```python
from build123d import *

# Parameters (mm, degrees)
BOSS_EXTRUDE1_DEPTH = 10
FILLET1_R           = 10
FILLET2_R           = 10


with BuildPart() as part:
    # Sketch2 → Boss-Extrude1 (new body)
    with BuildSketch(Plane.XY):
        Polygon((-10.989010989, 64.197802198), (29.010989011, 64.197802198), (29.010989011, -37.802197802), (-5.989010989, -37.802197802), align=None)
    extrude(amount=BOSS_EXTRUDE1_DEPTH)

    # Fillet1
    # the kernel refuses this fillet: 10 mm, written as the material it takes off along each edge
    with BuildSketch(Plane(origin=(-35.989010989, 64.197802198, 0), x_dir=(0, 0, 1), z_dir=(1, 0, 0))) as fillet1_piece_1:
        with BuildLine():
            CenterArc((FILLET1_R, FILLET1_R), FILLET1_R, 180, 90)
            Line((0, FILLET1_R), (0, 0))
            Line((0, 0), (FILLET1_R, 0))
        make_face()
    extrude(amount=90, mode=Mode.SUBTRACT)
    with BuildSketch(Plane(origin=(-35.989010989, 64.197802198, 10), x_dir=(0, 0, -1), z_dir=(1, 0, 0))) as fillet1_piece_2:
        with BuildLine():
            CenterArc((FILLET1_R, -FILLET1_R), FILLET1_R, 90, 90)
            Line((0, -FILLET1_R), (0, 0))
            Line((0, 0), (FILLET1_R, 0))
        make_face()
    extrude(amount=90, mode=Mode.SUBTRACT)

    # Fillet2
    # the kernel refuses this fillet: 10 mm, written as the material it takes off along each edge
    with BuildSketch(Plane(origin=(54.010989011, -37.802197802, 0), x_dir=(0, 0, 1), z_dir=(-1, 0, 0)), Plane(origin=(54.010989011, -37.802197802, 10), x_dir=(0, 1, 0), z_dir=(-1, 0, 0))) as fillet2_piece_1:
        with BuildLine():
            CenterArc((FILLET2_R, FILLET2_R), FILLET2_R, 180, 90)
            Line((0, FILLET2_R), (0, 0))
            Line((0, 0), (FILLET2_R, 0))
        make_face()
    extrude(amount=85, mode=Mode.SUBTRACT)


solid = part.part
```
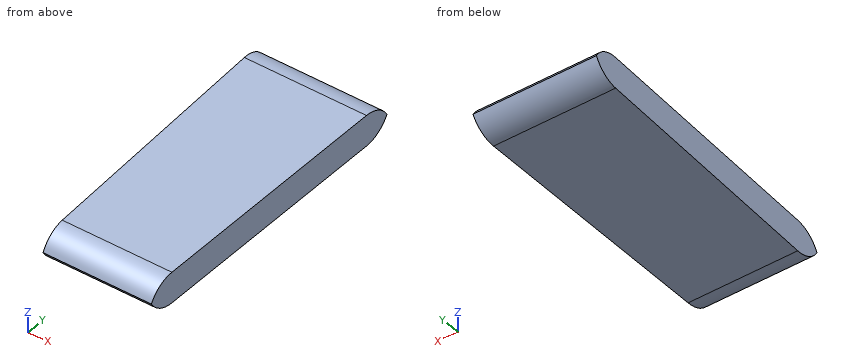
Can you work these out from the model? Positions are in its coordinate system, mm. Round coordinates to 2 decimals unless told otherwise and drop trailing zeros. Order: outer loops, then holes, each group sorted by start corner. A loop starts at its lowest first (then second) coordinate and runs counter-clockwise, first axis right, second up. Notation, with made-up numbers: (85.25, 61) -> (114.25, 61) arc R14 cw to (114.25, 66) -> close; hole circle Ø1 at (43.25, 58). An arc over 180 degrees is marked (long way). Return JSON: item names as keys, results as strings. Group by question number.
1. I need wall thicknesses on line 1 (X direction, y = 54.5, z = 3.5); line 2 (Y direction, x = 9, z = 2); line 3 (Y direction, x = 6, z = 3.75). Which ranges of each line are inside material? Lowest first, please. Write a range as [from, to].
2. Will these pins go through, and if not, where does the flat tip stop? pin 1 (4 mm diameter, centred on y = 0, z = 6.5, fed in from -X); pin 2 (1.5 mm diameter, centred on y = -16.5, z = 2.5, fed in from -X).
3. If we section it at B-B, the plane y = 28: Write out the boundary of the cut face in (x, z).
4. If we section it at C-C, the plane z = 3: Write out the boundary of the cut face in (x, y), then the cut area to 3 significant figures.
5. If we section it at A-A, the plane x = 26: Write out the boundary of the cut face in (y, z).
Output values:
{
 "1": {"line 1": "[-10.51, 29.01]", "line 2": "[-33.8, 60.2]", "line 3": "[-35.61, 62]"},
 "2": {"pin 1": "x = -7.94", "pin 2": "x = -7.07"},
 "3": {"outline": "(-9.21, 0) -> (29.01, 0) -> (29.01, 10) -> (-9.21, 10) -> close"},
 "4": {"outline": "(-10.85, 61.34) -> (-6.13, -34.94) -> (29.01, -34.94) -> (29.01, 61.34) -> close", "area": "3,610 mm²"},
 "5": {"outline": "(-36.46, 5) arc R10 ccw to (-27.8, 0) -> (54.2, 0) arc R10 ccw to (62.86, 5) arc R10 ccw to (54.2, 10) -> (-27.8, 10) arc R10 ccw to start"}
}
